Here's how the part is built. I have some questions about the finished solid (model axes, mm). Face numbers are marked on the shaded views. A direction names the side the tool comes from. Round coordinates to 2 decimals unless told otherwise and drop trailing zeros. Order: outer loops, then holes, each group sorted by start corner. A loop starts at its lowest first (then second) coordinate and runs counter-clockwise, first axis right, second up.
```python
from build123d import *

# Parameters (mm, degrees)
SKETCH1_W           = 100
SKETCH1_H           = 48
BOSS_EXTRUDE1_DEPTH = 7
CUT_EXTRUDE1_REACH  = 113.144
SKETCH2_R           = 3.2
SKETCH2_R_2         = 2.2
SKETCH3_W           = 100
SKETCH3_H           = 8
BOSS_EXTRUDE2_DEPTH = 10.2
SKETCH4_R           = 6.6
CUT_EXTRUDE2_DEPTH  = 5.25
SKETCH5_R           = 2.6
CUT_EXTRUDE3_DEPTH  = 0.1
SKETCH7_R           = 1.7
CUT_EXTRUDE4_DEPTH  = 113.233729333
CUT_EXTRUDE5_REACH  = 114.249
SKETCH8_R           = 1.7
CUT_EXTRUDE6_REACH  = 116.257
SKETCH9_W           = 3.3
SKETCH9_H           = 10.5
SKETCH10_R          = 3.2
BOSS_EXTRUDE3_DEPTH = 14
SHELL1_T            = 2.5
FILLET3_R           = 10


with BuildPart() as part:
    # Sketch1 → Boss-Extrude1 (new body)
    with BuildSketch(Plane.XY):
        with Locations((50, 24)):
            Rectangle(SKETCH1_W, SKETCH1_H)
    extrude(amount=BOSS_EXTRUDE1_DEPTH)

    # Sketch2 → Cut-Extrude1 (cut, up to next)
    with BuildSketch(Plane.XY.offset(7), mode=Mode.PRIVATE) as cut_extrude1_sk1:
        with Locations((15, 29)):
            Circle(SKETCH2_R)
    cut_extrude1_tool1 = extrude(cut_extrude1_sk1.sketch, amount=-CUT_EXTRUDE1_REACH, mode=Mode.PRIVATE) & part.part
    # Sketch2 → Cut-Extrude1 (cut, up to next)
    with BuildSketch(Plane.XY.offset(7), mode=Mode.PRIVATE) as cut_extrude1_sk2:
        with Locations((33.75, 29)):
            Circle(SKETCH2_R_2)
    cut_extrude1_tool2 = extrude(cut_extrude1_sk2.sketch, amount=-CUT_EXTRUDE1_REACH, mode=Mode.PRIVATE) & part.part
    # Sketch2 → Cut-Extrude1 (cut, up to next)
    with BuildSketch(Plane.XY.offset(7), mode=Mode.PRIVATE) as cut_extrude1_sk3:
        with Locations((55, 29)):
            Circle(SKETCH2_R_2)
    cut_extrude1_tool3 = extrude(cut_extrude1_sk3.sketch, amount=-CUT_EXTRUDE1_REACH, mode=Mode.PRIVATE) & part.part
    # Sketch2 → Cut-Extrude1 (cut, up to next)
    with BuildSketch(Plane.XY.offset(7), mode=Mode.PRIVATE) as cut_extrude1_sk4:
        with Locations((76.25, 29)):
            Circle(SKETCH2_R_2)
    cut_extrude1_tool4 = extrude(cut_extrude1_sk4.sketch, amount=-CUT_EXTRUDE1_REACH, mode=Mode.PRIVATE) & part.part
    add(cut_extrude1_tool1.solids().sort_by_distance((15, 29, 7))[0], mode=Mode.SUBTRACT)
    add(cut_extrude1_tool2.solids().sort_by_distance((33.75, 29, 7))[0], mode=Mode.SUBTRACT)
    add(cut_extrude1_tool3.solids().sort_by_distance((55, 29, 7))[0], mode=Mode.SUBTRACT)
    add(cut_extrude1_tool4.solids().sort_by_distance((76.25, 29, 7))[0], mode=Mode.SUBTRACT)

    # Sketch3 → Boss-Extrude2 (add)
    with BuildSketch(Plane(origin=(0, 0, 0), x_dir=(-1, 0, 0), z_dir=(0, 0, -1))):
        with Locations((-50, 4)):
            Rectangle(SKETCH3_W, SKETCH3_H)
    extrude(amount=BOSS_EXTRUDE2_DEPTH)

    # Sketch4 → Cut-Extrude2 (cut)
    with BuildSketch(Plane(origin=(0, 0, 0), x_dir=(-1, 0, 0), z_dir=(0, 0, -1))):
        with Locations((-76.25, 29)):
            Circle(SKETCH4_R)
        with Locations((-55, 29)):
            Circle(SKETCH4_R)
        with Locations((-33.75, 29)):
            Circle(SKETCH4_R)
    extrude(amount=-CUT_EXTRUDE2_DEPTH, mode=Mode.SUBTRACT)

    # Sketch5 → Cut-Extrude3 (cut)
    with BuildSketch(Plane.XY.offset(7)):
        with Locations((35.000022648, 4.052132501)):
            Circle(SKETCH5_R)
        with Locations((64.999977352, 4)):
            Circle(SKETCH5_R)
    extrude(amount=-CUT_EXTRUDE3_DEPTH, mode=Mode.SUBTRACT)

    # Sketch7 → Cut-Extrude4 (cut, through all)
    with BuildSketch(Plane.XY.offset(6.9)):
        with Locations((35.000022648, 4.052132501)):
            Circle(SKETCH7_R)
        with Locations((64.999977352, 4)):
            Circle(SKETCH7_R)
    extrude(amount=-CUT_EXTRUDE4_DEPTH, mode=Mode.SUBTRACT)

    # Sketch8 → Cut-Extrude5 (cut, up to next)
    with BuildSketch(Plane.XY.offset(7), mode=Mode.PRIVATE) as cut_extrude5_sk1:
        with Locations((10, 4.052132501)):
            Circle(SKETCH8_R)
    cut_extrude5_tool1 = extrude(cut_extrude5_sk1.sketch, amount=-CUT_EXTRUDE5_REACH, mode=Mode.PRIVATE) & part.part
    # Sketch8 → Cut-Extrude5 (cut, up to next)
    with BuildSketch(Plane.XY.offset(7), mode=Mode.PRIVATE) as cut_extrude5_sk2:
        with Locations((90, 4.052132501)):
            Circle(SKETCH8_R)
    cut_extrude5_tool2 = extrude(cut_extrude5_sk2.sketch, amount=-CUT_EXTRUDE5_REACH, mode=Mode.PRIVATE) & part.part
    add(cut_extrude5_tool1.solids().sort_by_distance((10, 4.052133, 7))[0], mode=Mode.SUBTRACT)
    add(cut_extrude5_tool2.solids().sort_by_distance((90, 4.052133, 7))[0], mode=Mode.SUBTRACT)


with BuildPart() as body_2:
    # Mirror1: mirrored copy
    add(part.part.mirror(Plane.XY.offset(-10.2)))

    # Sketch9 → Cut-Extrude6 (cut, up to next)
    with BuildSketch(Plane(origin=(100, 0, 0), x_dir=(0, 0, -1), z_dir=(1, 0, 0)), mode=Mode.PRIVATE) as cut_extrude6_sk1:
        with Locations((25.75, 5.25)):
            Rectangle(SKETCH9_W, SKETCH9_H)
    cut_extrude6_tool1 = extrude(cut_extrude6_sk1.sketch, amount=-CUT_EXTRUDE6_REACH, mode=Mode.PRIVATE) & body_2.part
    add(cut_extrude6_tool1.solids().sort_by_distance((100, 5.25, -25.75))[0], mode=Mode.SUBTRACT)


with BuildPart() as body_2_2:
    # Sketch10 → Boss-Extrude3 (new body)
    # profile 1 of 2: a face of its own
    with BuildSketch(Plane(origin=(0, 0, -27.4), x_dir=(-1, 0, 0), z_dir=(0, 0, -1))):
        with BuildLine():
            Line((-7.140610711, 38.2), (-22.859389289, 38.2))
            ThreePointArc((-22.859389289, 38.2), (-27.1, 29), (-22.859389289, 19.8))
            Line((-22.859389289, 19.8), (-7.140610711, 19.8))
            ThreePointArc((-7.140610711, 19.8), (-4.01117362, 23.934854908), (-2.9, 29))
            ThreePointArc((-2.9, 29), (-4.01117362, 34.065145092), (-7.140610711, 38.2))
        make_face()
        with Locations(Location((-15, 29, 0), (0, 0, 180))):
            Circle(SKETCH10_R, mode=Mode.SUBTRACT)
    # profile 2 of 2: a face of its own
    with BuildSketch(Plane(origin=(0, 0, -27.4), x_dir=(-1, 0, 0), z_dir=(0, 0, -1))):
        with Locations(Location((-15, 29, 0), (0, 0, 180))):
            Circle(SKETCH10_R)
    extrude(amount=BOSS_EXTRUDE3_DEPTH)

    # Shell1
    shell1_openings = [body_2_2.faces().sort_by_distance(p)[0] for p in [
        (15, 29, -27.4),
        (15, 29, -41.4),
    ]]
    offset(amount=SHELL1_T, openings=shell1_openings, kind=Kind.INTERSECTION)


with BuildPart() as body_2_1:
    add(body_2.part)

    # Combine1: union body 2 2
    add(body_2_2.part)

    # Fillet3
    fillet3_edges = [body_2_1.edges().sort_by_distance(p)[0] for p in [
        (0, 48, -23.9),
        (100, 48, -23.9),
    ]]
    fillet(fillet3_edges, radius=FILLET3_R)


solid = body_2_1.part
```
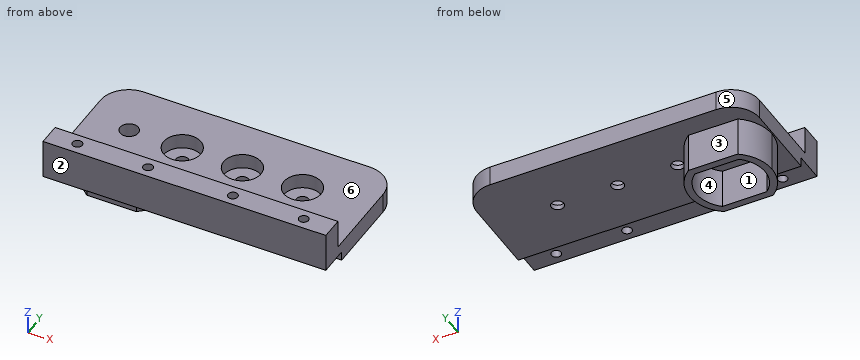
1) I need wall thicknesses on line 1 (Y direction, x = 55, z = -27); line 2 (X direction, y = 2.5, z = -20); line 3 (Y direction, x = 33.75, z = -23.1). Which ranges of each line are inside material? Lowest first, please.
2) If we section it at B-B (z = -36): Write out the boundary of the cut face in (x, y).
3) If we section it at D-D (y = 16): Write out the boundary of the cut face in (x, z).
4) For the marked faces 1, 2 and 3, which set-ups out of +Z, -Z, +X, -X, +Y, -Y let a thin tool reach every point of the face, with its end or its side?
5) If we section it at A-A (x = 76.25): Write out the boundary of the cut face in (y, z), plus the area to 3 significant figures.
6) If we section it at C-C (x = 15): Write out the boundary of the cut face in (y, z), plus the area to 3 significant figures.
7) We'd pull the mould along X, two halves only. Please class the marked faces 4, 5 and 6: +X half, -X half, draft (parallel to the pull), parting line (faces both ways), or undercut.
8) I'm going to push flat-ended pins straight in: pin 1 (11 mm diameter, centred on x = 13, z = -33.5, fed in from -Y); pin 2 (1.5 mm diameter, centred on y = 11, z = -29, fed in from -X); pin 3 (8 mm diameter, centred on x = 68, y = 30.5, fed in from +Z); pin 4 (5.5 mm diameter, centred on x = 33.75, y = 29, fed in from +Z). Where does each tip first touch, or does it pass through?
Solutions:
1. line 1: y = 10.5 to 26.8, 31.2 to 48
1. line 2: x = 0 to 9.31, 10.69 to 34.31, 35.69 to 64.2, 65.8 to 89.31, 90.69 to 100
1. line 3: y = 0 to 2.9, 5.2 to 22.4, 35.6 to 48
2. outline: (6.27, 17.3) - (23.73, 17.3) arc R14.6 ccw to (23.73, 40.7) - (6.27, 40.7) arc R14.6 ccw to start; hole (7.14, 19.8) - (22.86, 19.8) arc R12.1 ccw to (22.86, 38.2) - (7.14, 38.2) arc R12.1 ccw to start
3. outline: (0, -27.4) - (100, -27.4) - (100, -20.4) - (0, -20.4) - close
4. face 1: -Z
4. face 2: +Z, -Z, +X, -X, -Y
4. face 3: -Z, +X, -X, +Y
5. outline: (0, -24.1) - (10.5, -24.1) - (10.5, -27.4) - (26.8, -27.4) - (26.8, -25.65) - (22.4, -25.65) - (22.4, -20.4) - (8, -20.4) - (8, -10.2) - (0, -10.2) - close; (31.2, -27.4) - (48, -27.4) - (48, -20.4) - (35.6, -20.4) - (35.6, -25.65) - (31.2, -25.65) - close
5. area: 306 mm2
6. outline: (0, -24.1) - (10.5, -24.1) - (10.5, -27.4) - (17.3, -27.4) - (17.3, -41.4) - (19.8, -41.4) - (19.8, -27.4) - (25.8, -27.4) - (25.8, -20.4) - (8, -20.4) - (8, -10.2) - (0, -10.2) - close; (32.2, -27.4) - (38.2, -27.4) - (38.2, -41.4) - (40.7, -41.4) - (40.7, -27.4) - (48, -27.4) - (48, -20.4) - (32.2, -20.4) - close
6. area: 408 mm2
7. face 4: undercut
7. face 5: -X half
7. face 6: draft
8. pin 1: stops at y = 17.3
8. pin 2: passes through
8. pin 3: stops at z = -20.4
8. pin 4: stops at z = -25.65
